Check sheet for the modelled part. Datum: model origin and axes. Units: mm. Face numbers are marked on the shaded views. Give positions to 0.01 mm unless a question says otherwise; leave off trailing zeros. Order: outer loops, then holes, each group sorted by start corner. A loop starts at its lowest first (then second) coordinate and runs counter-clockwise, first axis right, second up. Notation, with made-up numbers: (79.25, 11) -> (126.25, 11) arc R15 ccw to (126.25, 36) -> close; hole circle Ø11 at (72, 50.5). An arc over 180 degrees is marked (long way). Answer in a Markdown table with one row per item. Add a question column.
(1) Go/stop test with flat-tipped pins: pin 1 (2.5 mm diameter, centred on x = 0, z = 1, fed in from -Y); pin 2 (1.4 mm diameter, centred on x = 12.5, z = -1, fed in from +Y); pin 3 (1.5 mm diameter, centred on x = -4.5, y = 2.5, fed in from -Z). Record where each tip stops, or that it passes through.
(2) Release check for a two-part mould opening along X. For the marked faces 1, 2 and 3 record: released by +X, released by -X, zero draft, split by the parting line, or undercut.
(3) Thickness scan on L1, parallel to Z at x = -13.55, y = 0.85; L2, parallel to Y at x = 6, z = 2; L3, parallel to Z at x = 0, y = 1.25. Record the ranges inside material, lowest first. Write a range as [from, to].
(4) Cross-section at C-C (y = 2.3). Record the cut outline in (x, z).
(5) Cross-section at B-B (z = 0.5). Record the cut outline in (x, y) (1 decimal), then the cut area to 3 significant figures.
(6) Cross-section at D-D (z = 3). Record the cut outline in (x, y).
(7) Cross-section at A-A (x = 0). Record the cut outline in (y, z), then the cut area to 3 significant figures.
Autodesk Inventor part; units mm, degrees
ref_plane "YZ Plane" through (0, 0, 0) normal (1, 0, 0) x (0, 1, 0)
ref_plane "XZ Plane" through (0, 0, 0) normal (0, 1, 0) x (-1, 0, 0)
sketch "Sketch1" plane through (0, 0, 0) normal (0, 1, 0) x (-1, 0, 0)
  circle A0 centre (0, 0) radius 3.45
  line L0 (0, 0) -> (-13.55, 0) construction
  line L1 (-0.0814, 2.4486) -> (-13.6164, 1.9989)
  line L2 (-13.6164, -1.9989) -> (-0.0814, -2.4486)
  arc A1 (-0.0814, -2.4486) -> (-0.0814, 2.4486) centre (0, 0) ccw
  arc A2 (-13.6164, 1.9989) -> (-13.6164, -1.9989) centre (-13.55, 0) ccw
  point P0 (-6.775, 0)
  point P1 (-15.55, 0)
  point P2 (3.45, 0)
  dimension "d0" = 6.9
  dimension "d2" = 4
  dimension "d3" = 1
  dimension "d4" = 19
extrude "Extrusion1" add sketch "Sketch1" along normal blind 1.4
extrude "Extrusion2" add sketch "Sketch1" along normal blind 3.7 contours A0 L2 A1 L1 | L1 A1 L2 A0
sketch "Sketch2" plane through (0, 3.7, 0) normal (0, 1, 0) x (1, 0, 0)
  circle A0 centre (0, 0) radius 3.45 construction
  circle A1 centre (0, 0) radius 1.2
  dimension "d9" = 2.4
extrude "Extrusion3" cut sketch "Sketch2" against normal through all
sketch "Sketch3" plane through (0, 3.7, 0) normal (0, 1, 0) x (1, 0, 0)
  circle A0 centre (0, 0) radius 3.45 construction
  circle A1 centre (0, 0) radius 2.3
  dimension "d12" = 4.6
extrude "Extrusion4" cut sketch "Sketch3" against normal blind 2
sketch "Sketch4" plane through (0, 0, 0) normal (0, -1, 0) x (1, 0, 0)
  arc A0 (2.509, 2.368) -> (2.509, -2.368) centre (0, 0) ccw construction
  circle A1 centre (0, 0) radius 2.35
  dimension "d15" = 1.1
extrude "Extrusion5" cut sketch "Sketch4" against normal blind 1
sketch "Sketch5" plane through (0, 0, 0) normal (0, -1, 0) x (1, 0, 0)
  arc A0 (13.6164, -1.9989) -> (13.6164, 1.9989) centre (13.55, 0) ccw construction
  line L0 (13.55, 0) -> (10.05, 0)
  line L1 (10.05, 0) -> (6.55, 0)
  line L2 (6.55, 0) -> (3.05, 0)
  point P0 (8.3, 0)
  point P1 (4.8, 0)
  point P2 (11.8, 0)
  point P3 (4.8, 0)
  dimension "d18" = 3.5
hole "Hole1" at (13.55, 0, 0) at (10.05, 0, 0) at (8.3, 0, 0) at (6.55, 0, 0) at (4.8, 0, 0) at (11.8, 0, 0) direction (0, 1, 0) diameter 0.3 end through all
mirror "Mirror1" about plane through (0, 0, 0) normal (1, 0, 0)
properties part number "SG90Horn2" material "PC/ABS Plastic"
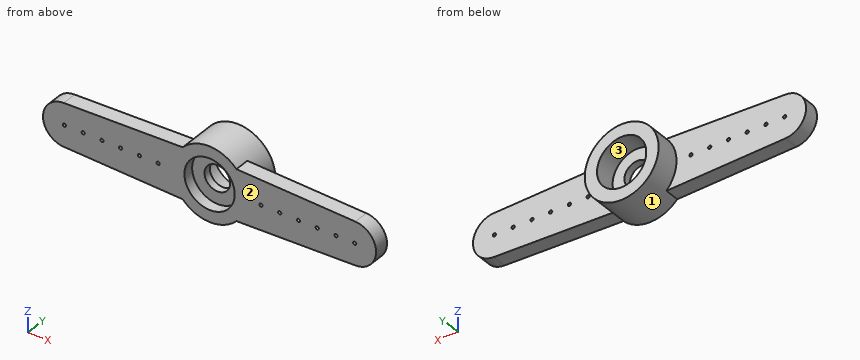
Answer below:
| question | item | result |
|---|---|---|
| 1 | pin 1 | stops at y = 1 |
| 1 | pin 2 | stops at y = 1.4 |
| 1 | pin 3 | passes through |
| 2 | face 1 | split by the parting line |
| 2 | face 2 | zero draft |
| 2 | face 3 | undercut |
| 3 | L1 | z = [-2, -0.15], [0.15, 2] |
| 3 | L2 | y = [0, 1.4] |
| 3 | L3 | z = [-3.45, -1.2], [1.2, 3.45] |
| 4 | outline | circle Ø6.9 at (0, 0); hole circle Ø4.6 at (0, 0) |
| 5 | outline | (-15.5, 0) -> (-2.3, 0) -> (-2.3, 1) -> (-1.1, 1) -> (-1.1, 1.7) -> (-2.2, 1.7) -> (-2.2, 3.7) -> (-3.4, 3.7) -> (-3.4, 1.4) -> (-15.5, 1.4) -> close; (1.1, 1) -> (2.3, 1) -> (2.3, 0) -> (15.5, 0) -> (15.5, 1.4) -> (3.4, 1.4) -> (3.4, 3.7) -> (2.2, 3.7) -> (2.2, 1.7) -> (1.1, 1.7) -> close |
| 5 | area | 44.0 mm² |
| 6 | outline | (-1.7, 0) -> (1.7, 0) -> (1.7, 3.7) -> (-1.7, 3.7) -> close |
| 7 | outline | (0, -3.45) -> (3.7, -3.45) -> (3.7, -2.3) -> (1.7, -2.3) -> (1.7, -1.2) -> (1, -1.2) -> (1, -2.35) -> (0, -2.35) -> close; (0, 2.35) -> (1, 2.35) -> (1, 1.2) -> (1.7, 1.2) -> (1.7, 2.3) -> (3.7, 2.3) -> (3.7, 3.45) -> (0, 3.45) -> close |
| 7 | area | 9.95 mm² |
